Input: dimensioned drawing with shaded views. Units: mm. Origin: part minimum x, y, z. A direction names the side the tool comes from. Coordinates: 2 decimals unless noted, no trailing zeros. Loops run counter-clockwise (first coordinate to the right, second up) from the corner with the lowest first, then second, coordinate; pieces in that order, holes last.
Item 1: Section query D-D, the plane z = 53.5. Return the cut outline in (x, y), then the cut area to 3 significant figures.
Item 2: Reachability of the marked faces 1, 2 and 3 from +Z, -Z, +X, -X, +Y, -Y: full face, straight path, thin tool, end or side. Return the list, or none.
Item 3: Section query B-B, the plane z = 12.5. Return the cut outline in (x, y), then the cut area to 3 significant figures.
Item 4: Section query A-A, the plane x = 4. Return the cut outline in (y, z), then the cut area to 3 significant figures.
Item 5: Pin query (flat end, axial travel): pin 1 Ø6 at (x, z) = (27.5, 21) entering from -Y; pin 2 Ø4 at (x, z) = (10, 7.5) entering from -Y; pin 3 Ø12 at (y, z) = (6, 30) entering from -X. Return the tip coordinate at first contact, or that it passes through.
Item 6: Section query C-C, the plane x = 20. Return the cut outline in (y, z).
Item 7: Pull-direction query (Z, two-part tool) for the marked faces 4, 5, 6 and 7; classes: +Z half, -Z half, draft (parallel to the pull), parting line (faces both ways), or undercut.
Item 8: Line query: probe 1 along Z at (x, y) = (32.5, 23); probe 2 along X at (y, z) = (14.75, 45.5); probe 3 along Z at (x, y) = (5.5, 16). Output: solid intervals per line, ascending.
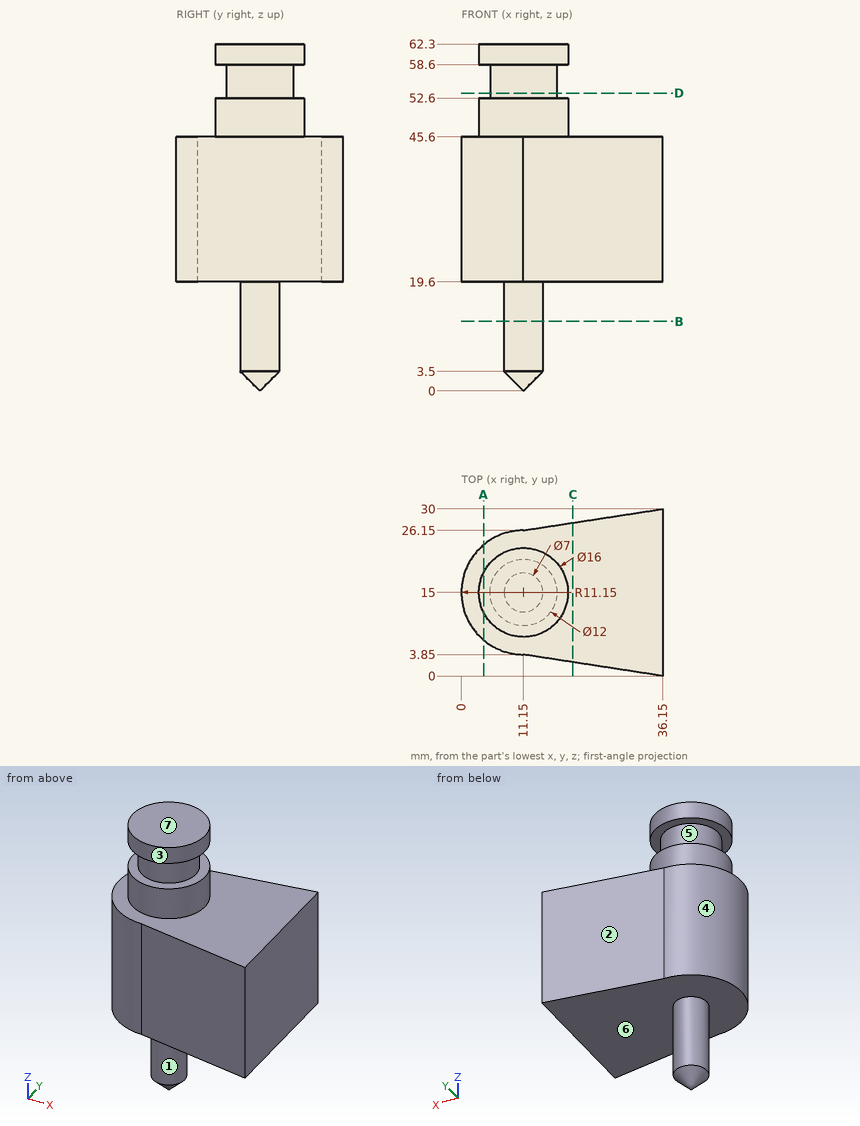
Verdict:
1. outline: circle Ø12 at (11.15, 15)
1. area: 113 mm2
2. face 1: -Z
2. face 2: +Z, -Z, -X, +Y
2. face 3: +Z
3. outline: circle Ø7 at (11.15, 15)
3. area: 38.5 mm2
4. outline: (6.44, 19.6) - (23.56, 19.6) - (23.56, 45.6) - (18.59, 45.6) - (18.59, 52.6) - (11.41, 52.6) - (11.41, 45.6) - (6.44, 45.6) - close; (11.41, 58.6) - (18.59, 58.6) - (18.59, 62.3) - (11.41, 62.3) - close
4. area: 522 mm2
5. pin 1: stops at y = 0.87
5. pin 2: stops at y = 11.5
5. pin 3: stops at x = 0.41
6. outline: (2.49, 19.6) - (27.51, 19.6) - (27.51, 45.6) - (2.49, 45.6) - close
7. face 4: draft
7. face 5: undercut
7. face 6: -Z half
7. face 7: +Z half
8. probe 1: z = 19.6 to 45.6
8. probe 2: x = 0 to 36.15
8. probe 3: z = 19.6 to 62.3
